Geometry: final body of the model. Coordinates: model frame, mm. A direction names the side the tool comes from. Coordinates: 2 decimals unless noted, no trailing zeros. Loops run counter-clockwise (first coordinate to the right, second up) from the corner with the lowest first, then second, coordinate; pieces in that order, holes last. Notation, with made-up numbers: (51, 84) - (64, 84) arc R30 cw to (64, 113) - close; hole circle Ø6 at (-33.75, 42). An arc over 180 degrees is marked (long way). Write each question's results on one line, items separated by ' | '. Start each with the question number.
Autodesk Inventor part; units mm, degrees
ref_plane "YZ Plane" through (0, 0, 0) normal (1, 0, 0) x (0, 1, 0)
ref_plane "XZ Plane" through (0, 0, 0) normal (0, 1, 0) x (-1, 0, 0)
ref_plane "XY Plane" through (0, 0, 0) normal (0, 0, 1) x (1, 0, 0)
sketch "Sketch2" plane through (0, 0, 0) normal (0, 0, 1) x (1, 0, 0)
  line L0 (0, 0) -> (-50.8, 0)
  line L1 (-101.6, 50.8) -> (-101.6, 1066.8)
  line L2 (-50.8, 1117.6) -> (50.8, 1117.6)
  arc A0 (-50.8, 1117.6) -> (-101.6, 1066.8) centre (-50.8, 1066.8) ccw
  arc A1 (-101.6, 50.8) -> (-50.8, 0) centre (-50.8, 50.8) ccw
  point P0 (0, 1117.6)
  dimension "d1" = 50.8
  dimension "d3" = 1016
  dimension "d6" = 101.6
  dimension "d7" = 101.6
  dimension "d8" = 50.8
  dimension "d9" = 1117.6
  dimension "d10" = 50.8
  dimension "d11" = 50.8
  dimension "d12" = 50.8
sketch "Sketch3" plane through (0, 0, 0) normal (1, 0, 0) x (0, 1, 0)
  circle A0 centre (0, 0) radius 27.94
  dimension "d13" = 55.88
sweep "Sweep1" add profiles "Sketch3" path "Sketch2"
shell "Shell1" thickness 2.54 removed faces 2 at (0, -1.1226, -9.2454) at (50.8, 1125.8465, -0.1295)
properties part number "connector2"
1) Access query for faces 1 (the flat face through (0, 25, 6)), 2 (the cylindrical face through (0.711, 1094.137, 9.728)), 3 (the cylindrical face through (-129.513, 565.912, -1.228)). Directions: +Z, -Z, +X, -X, +Y, -Y. A direction counts if a zero-diameter tool reaches every point of the face in a straight line with its end or side. Return the directions, or none.
2) Pull-direction query (X, two-part tool) for faces 4 (the cylindrical face through (-25.756, -5.506, 24.796)), 5 (the cylindrical face through (-77.373, 565.912, -7.629)), 6 (the flat face through (50.8, 1140.2, -12.3)); classes: released by +X, released by -X, zero draft, split by the parting line, or undercut.
3) Pin query (flat end, axial travel): pin 1 Ø12 at (x, y) = (-76, 323.5) entering from -Z; pin 2 Ø6 at (x, z) = (21, -16.5) entering from -Y; pin 3 Ø1 at (x, z) = (-18.5, -1.5) entering from +Y. Return the tip coordinate at first contact, or that it passes through.
4) Material intervals for line 1 (Y direction, x = -33, z = 0); line 2 (X direction, y = 206, z = 2); line 3 (Z direction, x = -22, y = 1117), sorted ascending. Write a range as [from, to].
5) Section query C-C on x = 26.5. Output: boundary loops of the cut face in (y, z).
6) Section query B-B on y = 653. Output: boundary loops of the cut face in (x, z), and give its area (3 significant figures).
7) Section query A-A on z = 0. Output: boundary loops of the cut face in (x, y).
Returned:
1) face 1: +Z, -Z, +X, -Y | face 2: +X | face 3: none
2) face 4: zero draft | face 5: undercut | face 6: released by +X
3) pin 1: stops at z = -19.91 | pin 2: stops at y = 1093.14 | pin 3: stops at y = 1145.52
4) line 1: y = [-27.94, -25.4], [25.4, 27.94], [1089.66, 1092.2], [1143, 1145.54] | line 2: x = [-129.47, -126.92], [-76.28, -73.73] | line 3: z = [-27.93, -25.39], [25.39, 27.93]
5) outline: circle Ø55.88 at (1117.6, 0); hole circle Ø50.8 at (1117.6, 0)
6) outline: circle Ø55.88 at (-101.6, 0); hole circle Ø50.8 at (-101.6, 0) | area: 426 mm²
7) outline: (-129.54, 50.8) arc R78.74 ccw to (-50.8, -27.94) - (0, -27.94) - (0, -25.4) - (-50.8, -25.4) arc R76.2 cw to (-127, 50.8) - (-127, 1066.8) arc R76.2 cw to (-50.8, 1143) - (50.8, 1143) - (50.8, 1145.54) - (-50.8, 1145.54) arc R78.74 ccw to (-129.54, 1066.8) - close; (-76.2, 50.8) arc R25.4 ccw to (-50.8, 25.4) - (0, 25.4) - (0, 27.94) - (-50.8, 27.94) arc R22.86 cw to (-73.66, 50.8) - (-73.66, 1066.8) arc R22.86 cw to (-50.8, 1089.66) - (50.8, 1089.66) - (50.8, 1092.2) - (-50.8, 1092.2) arc R25.4 ccw to (-76.2, 1066.8) - close
